```python
from build123d import *

# Parameters (mm, degrees)
BASE_FLANGE1_START = -2
BASE_FLANGE1_DEPTH = 2
SKETCH8_R          = 2
CUT_EXTRUDE1_DEPTH = 2


# Read off the part's stored shape, not the designer's step: Base-Flange1
with BuildPart() as part:
    # Base-Flange1 outline → Base-Flange1 (new body)
    with BuildSketch(Plane(origin=(0, 0, 0), x_dir=(1, 0, 0), z_dir=(0, 1, 0)).offset(BASE_FLANGE1_START)):
        with BuildLine():
            ThreePointArc((-29.187643745, 3.176759435), (-22.95, 7), (-16.712356255, 3.176759435))
            ThreePointArc((-16.712356255, 3.176759435), (-11.475, 1.832537182), (-6.237643745, 3.176759435))
            ThreePointArc((-6.237643745, 3.176759435), (0, 7), (6.237643745, 3.176759435))
            ThreePointArc((6.237643745, 3.176759435), (11.475, 1.832537182), (16.712356255, 3.176759435))
            ThreePointArc((16.712356255, 3.176759435), (22.95, 7), (29.187643745, 3.176759435))
            Line((29.187643745, 3.176759435), (29.187643745, 25.875))
            Line((29.187643745, 25.875), (-19.187643745, 25.875))
            Line((-19.187643745, 25.875), (-19.187643745, 50.875))
            Line((-19.187643745, 50.875), (-29.187643745, 50.875))
            Line((-29.187643745, 50.875), (-29.187643745, 3.176759435))
        make_face()
    extrude(amount=BASE_FLANGE1_DEPTH)

    # Sketch8 → Cut-Extrude1 (cut)
    with BuildSketch(Plane(origin=(0, 0, 0), x_dir=(1, 0, 0), z_dir=(0, 1, 0))):
        with Locations(Location((-24.187643745, 44.375, 0), (0, 0, 270))):
            Circle(SKETCH8_R)
        with Locations(Location((-24.187643745, 34.875, 0), (0, 0, 270))):
            Circle(SKETCH8_R)
    extrude(amount=-CUT_EXTRUDE1_DEPTH, mode=Mode.SUBTRACT)


solid = part.part
```
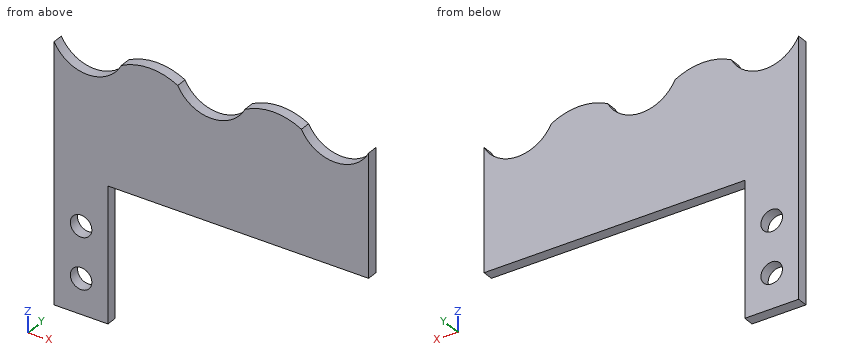
CAD build for the part. Positions are in the model's coordinates, mm. Coordinates: 2 decimals unless noted, no trailing zeros. Write each loop counter-clockwise with the first axis right and the second up, starting at its lowest first coordinate (ties: lowest second). Pieces come first, ordered by that corner, then holes.
(1) Cut at A-A, the plane y = -1.35. List the corners of the cut face in (x, z) (3 decimals).
(2) Cut at C-C, the plane z = -44. List the corners of the cut face in (x, y), and give its area (3 significant figures).
(3) Cut at D-D, the plane x = -15. List the corners of the cut face in (y, z) (3 decimals), and give its area (3 significant figures).
(4) Cut at B-B, the plane z = -5. List the corners of the cut face in (x, y).
(5) Flat gauge pin, fed straight in: pin 1 (1 mm diameter, centred on x = 21, y = -1, fed in from -Z) (3 decimals). Where does the tip first touch, or does it go through?
(6) Drill centre lines: probe 1 along X at (y, z) = (-0.75, -36); probe 2 along Z at (x, y) = (9.5, -1.55) (3 decimals); probe 3 along Z at (x, y) = (-11, -1.85) (3 decimals). Where is each one in solid material? Low to high.
Geometry says:
1. outline: (-29.188, -50.875) - (-19.188, -50.875) - (-19.188, -25.875) - (29.188, -25.875) - (29.188, -3.177) arc R7 cw to (16.712, -3.177) arc R10.875 ccw to (6.238, -3.177) arc R7 cw to (-6.238, -3.177) arc R10.875 ccw to (-16.712, -3.177) arc R7 cw to (-29.188, -3.177) - close; hole circle Ø4 at (-24.188, -44.375); hole circle Ø4 at (-24.188, -34.875)
2. outline: (-29.19, -2) - (-26.15, -2) - (-26.15, 0) - (-29.19, 0) - close; (-22.22, -2) - (-19.19, -2) - (-19.19, 0) - (-22.22, 0) - close
2. area: 12.1 mm2
3. outline: (-2, -25.875) - (0, -25.875) - (0, -2.42) - (-2, -2.42) - close
3. area: 46.9 mm2
4. outline: (-29.19, -2) - (-27.85, -2) - (-27.85, 0) - (-29.19, 0) - close; (-18.05, -2) - (-4.9, -2) - (-4.9, 0) - (-18.05, 0) - close; (4.9, -2) - (18.05, -2) - (18.05, 0) - (4.9, 0) - close; (27.85, -2) - (29.19, -2) - (29.19, 0) - (27.85, 0) - close
5. pin 1: stops at z = -25.875
6. probe 1: x = -29.19 to -25.84, -22.53 to -19.19
6. probe 2: z = -25.875 to -2.013
6. probe 3: z = -25.875 to -1.843
